from build123d import *

# Parameters (mm, degrees)
F1_DEPTH = 25.4
F2_R     = 5.08
F3_R     = 7.9375
F4_DEPTH = 25.4
F5_R     = 7.9375
F6_DEPTH = 25.4


with BuildPart() as f1:
    # F0 (on Front) → F1 (new body, symmetric)
    with BuildSketch(Plane.XZ):
        Polygon((-38.1, -38.1), (38.1, -38.1), (38.1, -31.6738), (-31.75, -31.6738), (-31.75, 38.1), (-38.1, 38.1), align=None)
    extrude(amount=F1_DEPTH, both=True)

    # F2
    f2_edges = [f1.edges().sort_by_distance(p)[0] for p in [
        (-31.75, 0, 38.1),
        (-31.75, 0, -31.6738),
        (38.1, 0, -31.6738),
    ]]
    fillet(f2_edges, radius=F2_R)

    # F3 (on face) → F4 (cut)
    with BuildSketch(Plane(origin=(-38.1, 0, 0), x_dir=(0, -1, 0), z_dir=(-1, 0, 0))):
        with Locations((0, 11.1125)):
            Circle(F3_R)
    extrude(amount=-F4_DEPTH, mode=Mode.SUBTRACT)

    # F5 (on face) → F6 (cut)
    with BuildSketch(Plane(origin=(0, 0, -38.1), x_dir=(1, 0, 0), z_dir=(0, 0, -1))):
        with Locations((11.1125, 0)):
            Circle(F5_R)
    extrude(amount=-F6_DEPTH, mode=Mode.SUBTRACT)


solid = f1.part
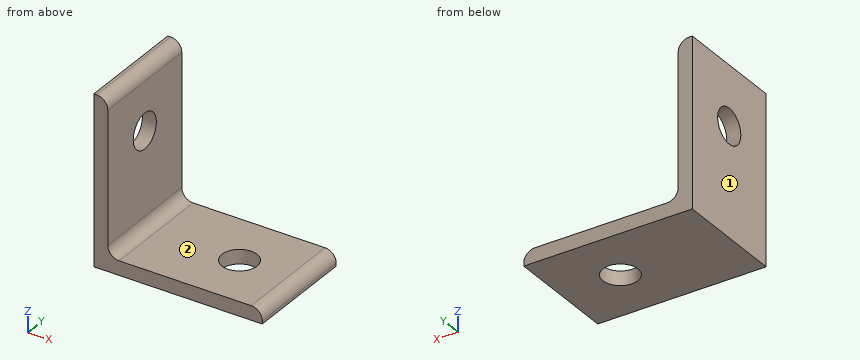
Input: part model. Units: mm. Frame: model coordinates. Face numbers are marked on the shaded views. A direction names the side the tool comes from. Give positions to 0.01 mm unless a question says otherwise; leave off trailing zeros. Order: outer loops, then holes, each group sorted by start corner. A loop starts at its lowest first (then second) coordinate and runs counter-clockwise, first axis right, second up. Notation, with made-up numbers: (-1, 38) -> (18, 38) arc R16 ccw to (18, 45) -> close; hole circle Ø1 at (-34, -10.5). An arc over 180 degrees is marked (long way). Use one line per item in the form item = value.
1) Section B-B, the plane x = 13. Return loops of the section in (y, z).
Response values:
outline = (-25.4, -38.1) -> (-7.71, -38.1) -> (-7.71, -31.67) -> (-25.4, -31.67) -> close; (7.71, -38.1) -> (25.4, -38.1) -> (25.4, -31.67) -> (7.71, -31.67) -> close
2) Line query: probe 1 along Z at (x, y) = (-20, 1); probe 2 along X at (y, z) = (-11, 14.5); probe 3 along Z at (x, y) = (-35, 0) (3 decimals). Output: solid intervals per line, ascending.
Response values:
probe_1 = -38.1 to -31.67
probe_2 = -38.1 to -31.75
probe_3 = -38.1 to 3.175, 19.05 to 37.759
3) First-contact query: pin 1 Ø8 at (y, z) = (-20, 13) entering from +X; pin 2 Ø9.5 at (x, y) = (11.11, 0) entering from -Z; pin 3 Ø12 at (x, y) = (-24, 16) entering from +Z; pin 4 Ø2 at (x, y) = (-10.5, 15.5) entering from +Z. Flat tips, straight axial feed; report the tip coordinate or a pass-through.
Response values:
pin_1 = -31.75
pin_2 = through
pin_3 = -30.43
pin_4 = -31.67
4) Reachability of the marked faces 1 and 2 from +Z, -Z, +X, -X, +Y, -Y: full face, straight path, thin tool, end or side. Return the list, or none.
Response values:
face_1 = +Z, -Z, -X, +Y, -Y
face_2 = +Z, +X, +Y, -Y
5) Section C-C, the plane y = 11. Return loops of the section in (x, z).
Response values:
outline = (-38.1, -38.1) -> (38.1, -38.1) -> (38.1, -36.75) arc R5.08 ccw to (33.02, -31.67) -> (-26.67, -31.67) arc R5.08 cw to (-31.75, -26.59) -> (-31.75, 33.02) arc R5.08 ccw to (-36.83, 38.1) -> (-38.1, 38.1) -> close
6) Section A-A, the plane y = 0. Return loops of the section in (x, z) (3 decimals), and give its area (3 significant figures).
Response values:
outline = (-38.1, -38.1) -> (3.175, -38.1) -> (3.175, -31.674) -> (-26.67, -31.674) arc R5.08 cw to (-31.75, -26.594) -> (-31.75, 3.175) -> (-38.1, 3.175) -> close; (-38.1, 19.05) -> (-31.75, 19.05) -> (-31.75, 33.02) arc R5.08 ccw to (-36.83, 38.1) -> (-38.1, 38.1) -> close; (19.05, -38.1) -> (38.1, -38.1) -> (38.1, -36.754) arc R5.08 ccw to (33.02, -31.674) -> (19.05, -31.674) -> close
area = 724 mm^2
7) Section D-D, the plane z = 15. Return loops of the section in (x, y).
Response values:
outline = (-38.1, -25.4) -> (-31.75, -25.4) -> (-31.75, -6.92) -> (-38.1, -6.92) -> close; (-38.1, 6.92) -> (-31.75, 6.92) -> (-31.75, 25.4) -> (-38.1, 25.4) -> close
